Check sheet for the modelled part. Datum: model origin and axes. Units: mm. A direction names the side the tool comes from. Give positions to 0.01 mm unless a question says otherwise; leave off trailing zeros. Loops run counter-clockwise (first coordinate to the right, second up) from the corner with the lowest first, then second, coordinate; pieces in that order, holes last. Notation, with made-up numbers: (-20, 80.5) - (14, 80.5) arc R21 cw to (14, 101.5) - close; hole circle Ø6 at (36.25, 5). An arc over 180 degrees is marked (long way). Use CSV: the item, a comma, the result in double quotes.
from build123d import *

# Parameters (mm, degrees)
F0_W      = 22.5
F0_H      = 12.65
F1_DEPTH  = 23
F2_W      = 12.65
F2_H      = 2.7
F3_DEPTH  = 5
F4_W      = 4
F4_H      = 1.5
F5_DEPTH  = 3
F6_R      = 1.25
F7_DEPTH  = 2.7
F8_W      = 12.65
F8_H      = 2.7
F9_DEPTH  = 5
F10_R     = 1.25
F11_DEPTH = 2.7
F12_R     = 2.375
F13_DEPTH = 4
F14_R     = 2.375
F15_DEPTH = 2.75
F17_DEPTH = 2.7
F19_DEPTH = 2.7


with BuildPart() as f1:
    # F0 (on Top) → F1 (new body)
    with BuildSketch(Plane.XY):
        Rectangle(F0_W, F0_H)
    extrude(amount=F1_DEPTH)

    # F2 (on face) → F3 (join)
    with BuildSketch(Plane(origin=(-11.25, 0, 0), x_dir=(0, -1, 0), z_dir=(-1, 0, 0))):
        with Locations((0, 17.35)):
            Rectangle(F2_W, F2_H)
    extrude(amount=F3_DEPTH)

    # F4 (on face) → F5 (join)
    with BuildSketch(Plane(origin=(-11.25, 0, 0), x_dir=(0, -1, 0), z_dir=(-1, 0, 0))):
        with Locations((0, 4.75)):
            Rectangle(F4_W, F4_H)
    extrude(amount=F5_DEPTH)

    # F6 (on face) → F7 (cut, through all)
    with BuildSketch(Plane.XY.offset(18.7)):
        with Locations((-14.0213416889, 0)):
            Circle(F6_R)
    extrude(amount=-F7_DEPTH, mode=Mode.SUBTRACT)

    # F8 (on face) → F9 (join)
    with BuildSketch(Plane.YZ.offset(11.25)):
        with Locations((0, 17.35)):
            Rectangle(F8_W, F8_H)
    extrude(amount=F9_DEPTH)

    # F10 (on face) → F11 (cut, through all)
    with BuildSketch(Plane.XY.offset(18.7)):
        with Locations((13.8043416664, 0)):
            Circle(F10_R)
    extrude(amount=-F11_DEPTH, mode=Mode.SUBTRACT)

    # F12 (on face) → F13 (join)
    with BuildSketch(Plane.XY.offset(23)):
        with BuildLine():
            ThreePointArc((-0.3125, -2.4803918541), (2.5, 0), (-0.3125, 2.4803918541))
            ThreePointArc((-0.3125, 2.4803918541), (-6.7716868718, 5.607612014), (-11.25, 0))
            ThreePointArc((-11.25, 0), (-6.7716868718, -5.607612014), (-0.3125, -2.4803918541))
        make_face()
        with Locations((-5.5, 0)):
            Circle(F12_R, mode=Mode.SUBTRACT)
        with Locations((-5.5, 0)):
            Circle(F12_R)
    extrude(amount=F13_DEPTH)

    # F14 (on face) → F15 (join)
    with BuildSketch(Plane.XY.offset(27)):
        with Locations((-5.5, 0)):
            Circle(F14_R)
    extrude(amount=F15_DEPTH)

    # F16 (on face) → F17 (cut, through all)
    with BuildSketch(Plane.XY.offset(18.7)):
        with BuildLine():
            Line((16.25, 0.75), (14.8043416664, 0.75))
            ThreePointArc((14.8043416664, 0.75), (14.990195789, 0.3952847075), (15.0543416664, 0))
            ThreePointArc((15.0543416664, 0), (14.990195789, -0.3952847075), (14.8043416664, -0.75))
            Line((14.8043416664, -0.75), (16.25, -0.75))
            Line((16.25, -0.75), (16.25, 0.75))
        make_face()
    extrude(amount=-F17_DEPTH, mode=Mode.SUBTRACT)

    # F18 (on face) → F19 (cut, through all)
    with BuildSketch(Plane.XY.offset(18.7)):
        with BuildLine():
            Line((-15.0213416889, 0.75), (-16.25, 0.75))
            Line((-16.25, 0.75), (-16.25, -0.75))
            Line((-16.25, -0.75), (-15.0213416889, -0.75))
            ThreePointArc((-15.0213416889, -0.75), (-15.2713416889, 0), (-15.0213416889, 0.75))
        make_face()
    extrude(amount=-F19_DEPTH, mode=Mode.SUBTRACT)


solid = f1.part
1. Go/stop test with flat-tipped pins: pin 1 Ø2 at (x, y) = (13.8, 0) entering from -Z; pin 2 Ø4 at (x, y) = (-14, 0) entering from -Z; pin 3 Ø1.3 at (y, z) = (-2.5, 21) entering from +X; pin 4 Ø3 at (x, y) = (-14.02, 0) entering from +Z. Record where each tip stops, or that it passes through.
Completed:
pin 1,"passes through"
pin 2,"stops at z = 4"
pin 3,"stops at x = 11.25"
pin 4,"stops at z = 18.7"
2. Sectioned sample at C-C, the plane z = 10. Record the boundary of the cut face in (x, y) (3 decimals).
Completed:
outline,"(-11.25, -6.325) - (11.25, -6.325) - (11.25, 6.325) - (-11.25, 6.325) - close"
3. Sectioned sample at A-A, the plane x = -5.5. Record the boundary of the cut face in (y, z) (3 decimals).
Completed:
outline,"(-6.325, 0) - (6.325, 0) - (6.325, 23) - (5.75, 23) - (5.75, 27) - (2.375, 27) - (2.375, 29.75) - (-2.375, 29.75) - (-2.375, 27) - (-5.75, 27) - (-5.75, 23) - (-6.325, 23) - close"
4. Sectioned sample at B-B, the plane y = -4. Record the boundary of the cut face in (x, z).
Completed:
outline,"(-16.25, 16) - (-11.25, 16) - (-11.25, 0) - (11.25, 0) - (11.25, 16) - (16.25, 16) - (16.25, 18.7) - (11.25, 18.7) - (11.25, 23) - (-1.37, 23) - (-1.37, 27) - (-9.63, 27) - (-9.63, 23) - (-11.25, 23) - (-11.25, 18.7) - (-16.25, 18.7) - close"
5. Scan lines: line 1 along Z through (x, y) = (-3, 3.5); line 2 along X through (y, z) = (0, 17.6); line 3 along Z through (x, y) = (-8, -5.5). Record each from-to range of solid material in increasing order.
Completed:
line 1,"z = 0 to 27"
line 2,"x = -12.77 to 12.55"
line 3,"z = 0 to 23"
6. Set-up check for faces 4 (the face through (11.25, 0, 8)), 5 (the face through (-14.25, 0, 5)), 6 (the face through (-13, 2, 5)), 7 (the face through (16, -0.75, 17)): record each of +Z, -Z, +X, -X, +Y, -Y from which the full face is reachable in a straight line by a thin tool's end or side.
Completed:
face 4,"-Z, +X, +Y, -Y"
face 5,"-Z, -X, +Y, -Y"
face 6,"-Z, -X, +Y"
face 7,"+Z, -Z, +X"
7. Release check for a two-part mould opening along Z. For faces 1 (the face through (16.25, -4, 17)), 2 (the face through (-13, 0, 5.5)), 3 (the face through (-2.9, 0.1, 27)) record: released by +Z, released by -Z, zero draft, split by the parting line, or undercut.
Completed:
face 1,"zero draft"
face 2,"undercut"
face 3,"released by +Z"
8. Sectioned sample at D-D, the plane x = 1.5. Record the boundary of the cut face in (y, z) (3 decimals), and give its area (3 significant figures).
Completed:
outline,"(-6.325, 0) - (6.325, 0) - (6.325, 23) - (2, 23) - (2, 27) - (-2, 27) - (-2, 23) - (-6.325, 23) - close"
area,"307 mm²"
